from build123d import *

# Parameters (mm, degrees)
EXTRUDE_THIN1_DEPTH = 460.375
SKETCH3_R           = 3.175
CUT_EXTRUDE1_DEPTH  = 462.277209629
SKETCH4_R           = 3.111919631
CUT_EXTRUDE2_DEPTH  = 462.277209629


with BuildPart() as part:
    # Sketch1 → Extrude-Thin1 (new body)
    with BuildSketch(Plane(origin=(0, 0, 0), x_dir=(1, 0, 0), z_dir=(0, 1, 0))):
        Polygon((-24.9936, -7.8232), (-24.9936, 17.5768), (0.4064, 17.5768), (0.4064, 15.0368), (-22.4536, 15.0368), (-22.4536, -7.8232), align=None)
    extrude(amount=EXTRUDE_THIN1_DEPTH)

    # Sketch3 → Cut-Extrude1 (cut, through all)
    with BuildSketch(Plane(origin=(-22.4536, 0, 0), x_dir=(0, 0, -1), z_dir=(1, 0, 0))):
        with Locations((3.205834921, 371.475)):
            Circle(SKETCH3_R)
    extrude(amount=-CUT_EXTRUDE1_DEPTH, mode=Mode.SUBTRACT)

    # Sketch4 → Cut-Extrude2 (cut, through all)
    with BuildSketch(Plane(origin=(-22.4536, 0, 0), x_dir=(0, 0, -1), z_dir=(1, 0, 0))):
        with Locations((2.761783971, 8.89)):
            Circle(SKETCH4_R)
    extrude(amount=-CUT_EXTRUDE2_DEPTH, mode=Mode.SUBTRACT)


solid = part.part
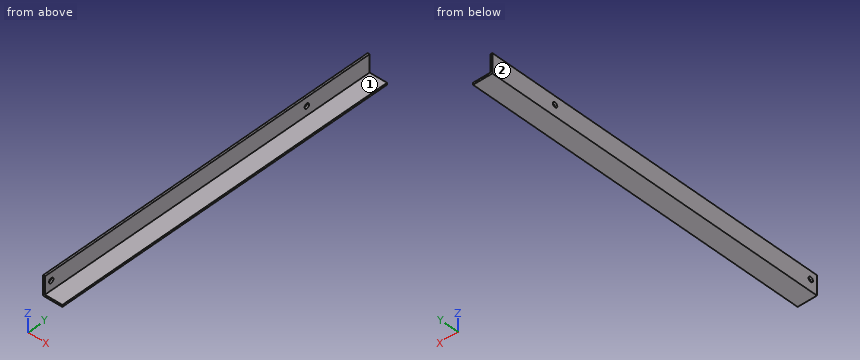
Can you work these out from the model? Positions are in its coordinate system, mm. Face numbers are marked on the shaded views. A direction names the side the tool comes from. Round coordinates to 2 decimals unless told otherwise and drop trailing zeros. Write each loop counter-clockwise with the first axis right and the second up, starting at its lowest first coordinate (ties: lowest second). Pieces come first, ordered by that corner, then holes. Notation, with made-up numbers: M 11.25,34 L 35.25,34 A22 cw 35.25,62 Z; hole C 77,48 d6. An arc over 180 degrees is marked long. Use a Markdown table: item, result.
Item 1: I want a section at A-A (z = -10.75). List the corners of the cut face in (x, y) for me (3 decimals).
Found:
| item | result |
|---|---|
| outline | M -24.994,0 L -22.454,0 L -22.454,460.375 L -24.994,460.375 Z |
Item 2: If I drill on line 1 along Z through (x, y) = (-14.75, 330); line 2 along X through (y, z) = (279, -4.5), over which ranges is the centre line in solid material (lowest first)? Write a range as [from, to].
Found:
| item | result |
|---|---|
| line 1 | z = [-17.58, -15.04] |
| line 2 | x = [-24.99, -22.45] |
Item 3: Which directions (+Z, -Z, +X, -X, +Y, -Y) give clear straight access to the entire face, cutting with the end or side of a thin tool? Please do the marked faces 1 and 2.
Found:
| item | result |
|---|---|
| face 1 | +Z, +X, +Y, -Y |
| face 2 | +Z, -Z, -X, +Y, -Y |
Item 4: For pin 1 Ø11.5 at (x, y) = (-16, 119) entering from +Z; pin 2 Ø11.5 at (y, z) = (116.5, 0.5) entering from +X, each with a flat end and sliding along its axis, tell me the tip position at first contact or that it passes through.
Found:
| item | result |
|---|---|
| pin 1 | stops at z = -15.04 |
| pin 2 | stops at x = -22.45 |
Item 5: I want a section at C-C (x = -12). List the corners of the cut face in (y, z) for me (3 decimals), and give its area (3 significant figures).
Found:
| item | result |
|---|---|
| outline | M 0,-17.577 L 460.375,-17.577 L 460.375,-15.037 L 0,-15.037 Z |
| area | 1,170 mm2 |
Item 6: I want a section at B-B (y = 235.5). List the corners of the cut face in (x, z) for me.
Found:
| item | result |
|---|---|
| outline | M -24.99,-17.58 L 0.41,-17.58 L 0.41,-15.04 L -22.45,-15.04 L -22.45,7.82 L -24.99,7.82 Z |
